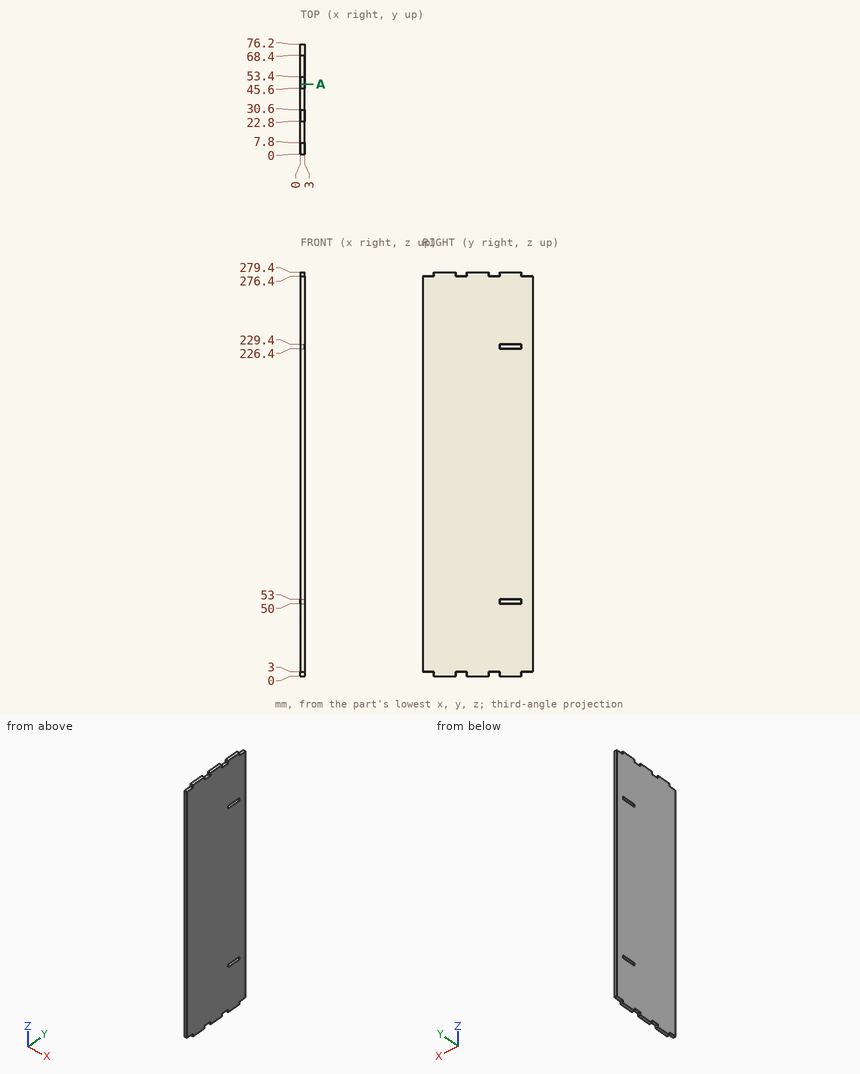
The drawing under review shows one solid part. Ordinate dimensions are in mm from its lowest x, y, z. Give positions to 0.01 mm unless a question says otherwise; leave off trailing zeros. Loops run counter-clockwise (first coordinate to the right, second up) from the corner with the lowest first, then second, coordinate; pieces in that order, holes last. Notation, with made-up numbers: M 8.25,47.5 L 46.25,47.5 A23 ccw 46.25,62.5 Z; hole C -30.5,60.25 d10. An arc over 180 degrees is marked long. Return JSON: item names as keys, results as strings. Group by question number.
Item 1: We need section A-A (y = 48.5). Give the boundary of the cut face in (x, z).
Item 2: For probe 1 along Z at (x, y) = (2.4, 65.5); probe 2 along Z at (x, y) = (2.95, 29.5), list the stretches that pass through material, from the lowest coordinate up.
Item 3: Insertion check: pin 1 Ø1.5 at (x, z) = (2, 1) entering from +Y; pin 2 Ø1.5 at (x, z) = (1.5, 277.5) entering from -Y. Each pin has a flat end and moves straight along its axis. Give the tip position at first contact, or say it passes through.
Output:
{
 "1": {"outline": "M 0,3 L 3,3 L 3,276.4 L 0,276.4 Z"},
 "2": {"probe 1": "z = 0 to 50, 53 to 226.4, 229.4 to 279.4", "probe 2": "z = 3 to 276.4"},
 "3": {"pin 1": "stops at y = 68.4", "pin 2": "stops at y = 7.8"}
}
